from build123d import *

# Parameters (mm, degrees)
SKETCH_W        = 15
SKETCH_H        = 35
PAD_DEPTH       = 15
SKETCH001_W     = 25
SKETCH001_H     = 36
SKETCH001_W_2   = 4.6
SKETCH001_H_2   = 4.6
SKETCH001_W_3   = 1.1
SKETCH001_H_3   = 4
POCKET_DEPTH    = 10
SKETCH002_W     = 4
SKETCH002_H     = 1.1
POCKET001_DEPTH = 10
SKETCH003_W     = 6
SKETCH003_H     = 6
POCKET002_DEPTH = 5.8


with BuildPart() as part:
    # Sketch → Pad (new body)
    with BuildSketch(Plane.XY):
        with Locations((63.25, -96.5)):
            Rectangle(SKETCH_W, SKETCH_H)
    extrude(amount=PAD_DEPTH)

    # Sketch001 (on DatumPlane) → Pocket (cut)
    with BuildSketch(Plane.XY.offset(15)):
        with Locations((62.5, -102)):
            Rectangle(SKETCH001_W, SKETCH001_H)
        with Locations((63.25, -96.5)):
            Rectangle(SKETCH001_W_2, SKETCH001_H_2, mode=Mode.SUBTRACT)
        with Locations((63.25, -96.5)):
            Rectangle(SKETCH001_W_3, SKETCH001_H_3)
    extrude(amount=-POCKET_DEPTH, mode=Mode.SUBTRACT)

    # Sketch002 (on DatumPlane) → Pocket001 (cut)
    with BuildSketch(Plane.XY.offset(15)):
        with Locations((63.25, -96.5)):
            Rectangle(SKETCH002_W, SKETCH002_H)
    extrude(amount=-POCKET001_DEPTH, mode=Mode.SUBTRACT)

    # Sketch003 (on DatumPlane) → Pocket002 (cut)
    with BuildSketch(Plane.XY.offset(15)):
        with Locations((63, -96)):
            Rectangle(SKETCH003_W, SKETCH003_H)
    extrude(amount=-POCKET002_DEPTH, mode=Mode.SUBTRACT)


solid = part.part
Work out the finished part from the listing and answer in its coordinate system (mm). A direction names the side the tool comes from. Round coordinates to 2 decimals unless told otherwise and drop trailing zeros. Order: outer loops, then holes, each group sorted by start corner. A loop starts at its lowest first (then second) coordinate and runs counter-clockwise, first axis right, second up. Notation, with made-up numbers: M 32,-3 L 77,-3 A15 cw 77,12 Z; hole C 33.5,67.25 d7. An arc over 180 degrees is marked long. Put each result on its own line as item: value. Start each with the question number.
Q1. Section B-B, the plane y = -95.5 is taken. Write down the section's boundary in (x, z).
Q2. Straight lines are drawn through the part: L1, parallel to Y at x = 62.5, z = 8.25; L2, parallel to Z at x = 60, y = -88; L3, parallel to Y at x = 58, z = 5.75. For each, find the intervals that lie inside material, in ascending order. Write a range as [from, to].
Q3. Section D-D, the plane z = 10 is taken. Write down the section's boundary in (x, y), and give its area (3 significant figures).
Q4. For a pull along X with two mould halves and no side action, classify faces 1 (the flat face through (65, -97.05, 7)), 2 (the flat face through (63.8, -95, 7)), 3 (the flat face through (60.95, -97, 7)), 4 (the flat face through (63, -114, 2)) as pulls with the +X half, pulls with the -X half, needs draft (parallel to the pull), parting line crosses it, or undercut.
Q5. Flat-ended cylindrical pins translate along their axes: pin 1 (4.5 mm diameter, centred on x = 63.5, y = -99, fed in from +Z); pin 2 (1.2 mm diameter, centred on y = -95.5, z = 8, fed in from +X); pin 3 (8 mm diameter, centred on x = 66, z = 9.5, fed in from -Y). Find the tip coordinate at first contact, or state that the pin passes through.
Q6. Section A-A, the plane z = 5.5 is taken. Write down the section's boundary in (x, y).
Q7. Section C-C, the plane x = 69 is taken. Write down the section's boundary in (y, z).
Q8. A tool of negligible diameter and unlimited length cuts with its end or side. For faces 5 (the flat face through (65, -95.95, 7)), 6 (the flat face through (63, -84, 10)), 7 (the flat face through (63, -79, 7)), 8 (the flat face through (63, -81, 15)), 9 (the flat face through (63, -98.8, 7)), from which of +Z, -Z, +X, -X, +Y, -Y can it reach the whole face along a straight path? Write none if from no direction.
Findings below:
1. outline: M 55.75,0 L 70.75,0 L 70.75,5 L 65.55,5 L 65.55,9.2 L 63.8,9.2 L 63.8,5 L 62.7,5 L 62.7,9.2 L 60.95,9.2 L 60.95,5 L 55.75,5 Z
2. L1: y = [-98.8, -97.05], [-95.95, -94.2], [-84, -79]
2. L2: z = [0, 5]
2. L3: y = [-84, -79]
3. outline: M 55.75,-84 L 70.75,-84 L 70.75,-79 L 55.75,-79 Z
3. area: 75.0 mm^2
4. face 1: undercut
4. face 2: undercut
4. face 3: pulls with the -X half
4. face 4: needs draft
5. pin 1: stops at z = 9.2
5. pin 2: stops at x = 65.55
5. pin 3: stops at y = -98.8
6. outline: M 55.75,-84 L 70.75,-84 L 70.75,-79 L 55.75,-79 Z; M 60.95,-98.8 L 65.55,-98.8 L 65.55,-94.2 L 60.95,-94.2 Z; hole M 61.25,-97.05 L 62.7,-97.05 L 62.7,-98.5 L 63.8,-98.5 L 63.8,-97.05 L 65.25,-97.05 L 65.25,-95.95 L 63.8,-95.95 L 63.8,-94.5 L 62.7,-94.5 L 62.7,-95.95 L 61.25,-95.95 Z
7. outline: M -114,0 L -79,0 L -79,15 L -84,15 L -84,5 L -114,5 Z
8. face 5: +Z
8. face 6: +Z, +X, -X
8. face 7: +Z, -Z, +X, -X, +Y
8. face 8: +Z, +X, -X, +Y, -Y
8. face 9: +Z, +X, -X, -Y
